```python
from build123d import *

# Parameters (mm, degrees)
EXTRUDE_SKETCH001_DEPTH = 1
SKETCH002_R             = 2.5
EXTRUDE_SKETCH002_DEPTH = 5
FILLET_R                = 2.4


with BuildPart() as sketch001_extrude:
    # Sketch001 → Extrude_Sketch001 (new body)
    with BuildSketch(Plane.XY):
        with BuildLine():
            ThreePointArc((2.5, 1.658312), (-3, 0), (2.5, -1.658312))
            Line((2.5, 1.658312), (2.5, -1.658312))
        make_face()
    extrude(amount=EXTRUDE_SKETCH001_DEPTH)


with BuildPart() as fusion:
    # Sketch002 → Extrude_Sketch002 (new body)
    with BuildSketch(Plane.XY.offset(1)):
        Circle(SKETCH002_R)
    extrude(amount=EXTRUDE_SKETCH002_DEPTH)

    # Fillet
    fillet_edges = [fusion.edges().sort_by_distance(p)[0] for p in [
        (-2.5, 0, 6),
    ]]
    fillet(fillet_edges, radius=FILLET_R)

    # Fusion: union Sketch001_Extrude
    add(sketch001_extrude.part)


solid = fusion.part
```
Verification items for the finished model (mm, model axes). A direction names the side the tool comes from. Give positions to 0.01 mm unless a question says otherwise; leave off trailing zeros. Loops run counter-clockwise (first coordinate to the right, second up) from the corner with the lowest first, then second, coordinate; pieces in that order, holes last. Notation, with made-up numbers: M -28.75,7.25 L -14.75,7.25 A17 cw -14.75,31.25 Z; hole C -18.5,-36 d11. An arc over 180 degrees is marked long. Return JSON: item names as keys, results as strings.
1) Section check A-A, the plane z = 2.5. Enter the section's corners in (x, y), and give its area (3 significant figures).
Findings:
{"outline": "C 0,0 d5", "area": "19.6 mm2"}
2) Material ranges on L1, parallel to Z at x = -1.15, y = 2.25; L2, parallel to Y at x = 0, z = 2.6; L3, parallel to Z at x = 0.45, y = -0.35, recorded low to high. Write a range as [from, to].
Findings:
{"L1": "z = [0, 1]", "L2": "y = [-2.5, 2.5]", "L3": "z = [0, 5.95]"}
3) Gauge pin test, flat ends, axial feed: P1, Ø2, axis at x = 1.5, y = 2, coming from the +Z side; P2, Ø1, axis at x = -2, z = 5, coming from the -Y side; P3, Ø1.5, axis at x = 1.5, z = 1, coming from the -Y side. Record the tip position at first contact, or that the pin passes through.
Findings:
{"P1": "stops at z = 5.55", "P2": "stops at y = -1.56", "P3": "stops at y = -2.9"}
4) Tool access check on faces 1 (the flat face through (-2, -2, 1)), 2 (the flat face through (0, 0, 0)). Record the directions out of +Z, -Z, +X, -X, +Y, -Y that give a thin tool (end or side, any length) a straight path to the whole face; none if there is none.
Findings:
{"face 1": "+Z", "face 2": "-Z, +X, -X, +Y, -Y"}
